```python
from build123d import *

# Parameters (mm, degrees)
F0_W     = 38.1
F0_H     = 38.1
F1_DEPTH = 634.38786
F2_R     = 5
F3_DEPTH = 25.4


with BuildPart() as f1:
    # F0 (on Front) → F1 (new body)
    with BuildSketch(Plane.XZ):
        with BuildLine():
            Line((15.980036, 28.785883), (-28.469964, 28.785883))
            ThreePointArc((-28.469964, 28.785883), (-30.715028, 27.855947), (-31.644964, 25.610883))
            Line((-31.644964, 25.610883), (-31.644964, -18.839117))
            ThreePointArc((-31.644964, -18.839117), (-30.715028, -21.084181), (-28.469964, -22.014117))
            Line((-28.469964, -22.014117), (15.980036, -22.014117))
            ThreePointArc((15.980036, -22.014117), (18.2251, -21.084181), (19.155036, -18.839117))
            Line((19.155036, -18.839117), (19.155036, 25.610883))
            ThreePointArc((19.155036, 25.610883), (18.2251, 27.855947), (15.980036, 28.785883))
        make_face()
        with Locations((-6.244964, 3.385883)):
            Rectangle(F0_W, F0_H, mode=Mode.SUBTRACT)
    extrude(amount=F1_DEPTH)

    # F2 (on face) → F3 (cut)
    with BuildSketch(Plane.XY.offset(28.785883)):
        with Locations((-15.769964, -25.4)):
            Circle(F2_R)
        with Locations((3.280036, -25.4)):
            Circle(F2_R)
        with Locations((-15.769964, -608.98786)):
            Circle(F2_R)
        with Locations((3.280036, -608.98786)):
            Circle(F2_R)
    extrude(amount=-F3_DEPTH, mode=Mode.SUBTRACT)


solid = f1.part
```
Verification items for the finished model (mm, model axes). A direction names the side the tool comes from. Round coordinates to 2 decimals unless told otherwise and drop trailing zeros. Order: outer loops, then holes, each group sorted by start corner. A loop starts at its lowest first (then second) coordinate and runs counter-clockwise, first axis right, second up. Notation, with made-up numbers: (-6.5, 17.5) -> (25.5, 17.5) arc R24 cw to (25.5, 28.5) -> close; hole circle Ø9 at (-34, -14.5). An arc over 180 degrees is marked (long way). Put each result on its own line as item: value. Start each with the question number.
(1) Tool access check on faces 5 (the face through (-25.295, -313, 3)), 6 (the face through (2.2, -613.87, 25.66)), 7 (the face through (-29, 0, 4)). Record the directions out of +Z, -Z, +X, -X, +Y, -Y that give a thin tool (end or side, any length) a straight path to the whole face; none if there is none.
(2) Depth check by flat-ended pin: pin 1 Ø13 at (x, y) = (3.28, -25.4) entering from +Z. Enter the tip coordinate at first touch or a pass-through.
(3) Section check A-A (y = -125). Enter the section's corners in (x, z) (3 decimals).
(4) Section check B-B (z = -6). Enter the section's corners in (x, y), then the cut area to 3 significant figures.
(5) Material ranges on line 1 along X through (y, z) = (-25, 26); line 2 along X through (y, z) = (-25, 25); line 3 along X through (y, z) = (-201, 17.5), recorded low to high.
(6) Draft check along Y on faces 1 (the face through (-29, -634.388, 4)), 2 (the face through (-20.765, -25.18, 25.655)), 3 (the face through (-7, -313, -22.014)), 4 (the face through (-16.85, -613.87, 25.66)). Enter one of: +Y half, -Y half, draft (parallel to the pull), parting line (faces both ways), or undercut.
Completed:
1. face 5: +Y, -Y
1. face 6: +Z
1. face 7: +Z, -Z, +X, -X, +Y
2. pin 1: stops at z = 28.79
3. outline: (-31.645, -18.839) arc R3.175 ccw to (-28.47, -22.014) -> (15.98, -22.014) arc R3.175 ccw to (19.155, -18.839) -> (19.155, 25.611) arc R3.175 ccw to (15.98, 28.786) -> (-28.47, 28.786) arc R3.175 ccw to (-31.645, 25.611) -> close; hole (-25.295, -15.664) -> (12.805, -15.664) -> (12.805, 22.436) -> (-25.295, 22.436) -> close
4. outline: (-31.64, -634.39) -> (-25.29, -634.39) -> (-25.29, 0) -> (-31.64, 0) -> close; (12.81, -634.39) -> (19.16, -634.39) -> (19.16, 0) -> (12.81, 0) -> close
4. area: 8,060 mm2
5. line 1: x = -31.62 to -20.75, -10.79 to -1.7, 8.26 to 19.13
5. line 2: x = -31.64 to -20.75, -10.79 to -1.7, 8.26 to 19.16
5. line 3: x = -31.64 to -25.29, 12.81 to 19.16
6. face 1: -Y half
6. face 2: undercut
6. face 3: draft
6. face 4: undercut
